The model under review builds one solid part; all positions refer to its coordinate system, in mm. A direction names the side the tool comes from. Coordinates: 2 decimals unless noted, no trailing zeros. Order: outer loops, then holes, each group sorted by start corner. A loop starts at its lowest first (then second) coordinate and runs counter-clockwise, first axis right, second up.
```python
from build123d import *

# Parameters (mm, degrees)
PAD012_DEPTH    = 6
SKETCH029_R     = 5.3
POCKET012_DEPTH = 6
SKETCH031_R     = 1.6
POCKET014_DEPTH = 5


with BuildPart() as part:
    # CopySketch029 → Pad012 (new body)
    with BuildSketch(Plane.YZ):
        with BuildLine():
            Line((69.62, -34.0739220052), (104.26, -20.95))
            Line((104.26, -20.95), (104.26, -75.95))
            Line((104.26, -75.95), (40.01, -64.8058991482))
            Line((40.01, -64.8058991482), (40.01, -44.4358991482))
            ThreePointArc((53.3737933734, -34.0739220052), (44.4834146169, -36.4066415985), (40.01, -44.4358991482))
            Line((53.3737933734, -34.0739220052), (69.62, -34.0739220052))
        make_face()
    extrude(amount=PAD012_DEPTH)

    # Sketch029 (on Face7 of Pad012) → Pocket012 (cut)
    with BuildSketch(Plane(origin=(0, 0, 0), x_dir=(0, 1, 0), z_dir=(-1, 0, 0))):
        with Locations((52.5, 44.25)):
            Circle(SKETCH029_R)
    extrude(amount=-POCKET012_DEPTH, mode=Mode.SUBTRACT)

    # Sketch031 (on Face4 of Pocket012) → Pocket014 (cut)
    with BuildSketch(Plane(origin=(0, 0, 0), x_dir=(0, 1, 0), z_dir=(-1, 0, 0))):
        with Locations((74.913826, 48.264923)):
            Circle(SKETCH031_R)
        with Locations((74.851181, 34.284763)):
            Circle(SKETCH031_R)
        with Locations((41.828423, 63.335484)):
            Circle(SKETCH031_R)
        with Locations((74.867561, 68.275307)):
            Circle(SKETCH031_R)
        with Locations((102.321861, 48.275112)):
            Circle(SKETCH031_R)
        with Locations((102.306999, 23.636881)):
            Circle(SKETCH031_R)
        with Locations((102.284668, 72.393417)):
            Circle(SKETCH031_R)
    extrude(amount=-POCKET014_DEPTH, mode=Mode.SUBTRACT)


with BuildPart() as part_1:
    # Body005 placement: moved
    add(part.part.moved(Location((87, 0, 0))))


solid = part_1.part
```
(1) Wall thickness on probe 1 along Z at (x, y) = (89.1, 74); probe 2 along Z at (x, y) = (90.95, 50); probe 3 along Y at (x, z) = (92.2, -43): over which ranges is each line inside the solid? List them lowest first.
A:
probe 1: z = -70.7 to -69.62, -66.93 to -49.58, -46.95 to -35.64, -32.93 to -32.41
probe 2: z = -66.54 to -48.92, -39.58 to -34.07
probe 3: y = 40.25 to 47.35, 57.65 to 104.26
(2) We need section B-B, the plane x = 90. Count the separate pieces of the cut face and the enclosed holes in it, and give its area (3 significant figures).
A:
separate pieces: 1
enclosed holes: 8
area: 2,390 mm2
(3) For pin 1 Ø1.5 at (x, z) = (92, -36.5) entering from -Y; pin 2 Ø2.5 at (y, z) = (102.28, -72.39) entering from -X; pin 3 Ø1.5 at (x, y) = (92, 84.5) entering from -Z, all flat-tipped, find the tip position at first contact; note any pin that passes through.
A:
pin 1: stops at y = 43.51
pin 2: stops at x = 92
pin 3: stops at z = -72.65
(4) Machinability: for faces 4 (the face through (90, 40.01, -55)), 5 (the face through (90, 61, -34.074)), 6 (the face through (89.46, 41.62, -64.92)), which of the approach directions +Z, -Z, +X, -X, +Y, -Y give a long, thin tool a straight path to every point of the face, cutting with its end or side? Answer none if there is none.
A:
face 4: +Z, -Z, +X, -X, -Y
face 5: +Z, +X, -X
face 6: -X
(5) Draft analysis for pull direction X (two halves, no side actions). For faces 1 (the face through (89.465, 100.686, -72.464)), 2 (the face through (93, 80, -48)), 3 (the face through (92, 42, -63)), state which applies: released by +X, released by -X, zero draft, split by the parting line, or undercut.
A:
face 1: zero draft
face 2: released by +X
face 3: released by -X
(6) We need section A-A, the plane y = 55.5. Write out the cut boundary in (x, z), and give its area (3 significant figures).
A:
outline: (87, -67.49) - (93, -67.49) - (93, -48.62) - (87, -48.62) - close; (87, -39.88) - (93, -39.88) - (93, -34.07) - (87, -34.07) - close
area: 148 mm2
(7) We need section C-C, the plane y = 75. Write out the cut boundary in (x, z).
A:
outline: (87, -70.87) - (93, -70.87) - (93, -32.04) - (87, -32.04) - (87, -32.69) - (92, -32.69) - (92, -35.88) - (87, -35.88) - (87, -46.67) - (92, -46.67) - (92, -49.86) - (87, -49.86) - (87, -66.68) - (92, -66.68) - (92, -69.87) - (87, -69.87) - close
(8) We need section D-D, the plane z = -29.5. Write out the cut boundary in (x, y), and give its area (3 significant figures).
A:
outline: (87, 81.69) - (93, 81.69) - (93, 104.26) - (87, 104.26) - close
area: 135 mm2
